Input: part model. Units: mm. Frame: model coordinates. Face numbers are marked on the shaded views. A direction names the side the tool comes from. Round coordinates to 2 decimals unless told otherwise and drop trailing zeros. Write each loop counter-clockwise with the first axis right and the second up, starting at its lowest first coordinate (ties: lowest second). Pieces come first, ordered by that corner, then holes. Notation, with made-up numbers: (-15, 54) - (13, 54) arc R12 ccw to (13, 76) - close; hole circle Ø7 at (52.5, 65). An arc over 180 degrees is marked (long way). One line per item, written item: value. Start each with the question number.
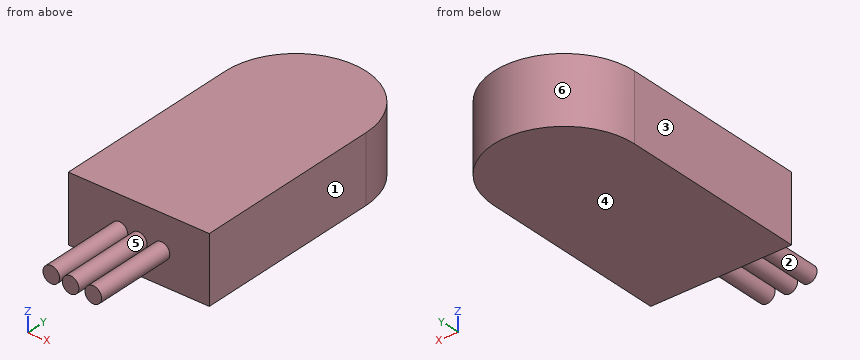
Autodesk Inventor part; units mm, degrees
ref_plane "YZ Plane" through (0, 0, 0) normal (1, 0, 0) x (0, 1, 0)
ref_plane "XZ Plane" through (0, 0, 0) normal (0, 1, 0) x (-1, 0, 0)
ref_plane "XY Plane" through (0, 0, 0) normal (0, 0, 1) x (1, 0, 0)
sketch "Sketch1" plane through (0, 0, 0) normal (0, 0, 1) x (1, 0, 0)
  line L0 (-8.5, 11.5) -> (8.5, 11.5)
  line L1 (8.5, 11.5) -> (8.5, -11.5)
  line L2 (8.5, -11.5) -> (-8.5, -11.5)
  line L3 (-8.5, -11.5) -> (-8.5, 11.5)
  line L4 (-8.5, 11.5) -> (8.5, -11.5) construction
  line L5 (8.5, 11.5) -> (-8.5, -11.5) construction
  arc A0 (8.5, 11.5) -> (-8.5, 11.5) centre (0, 11.5) ccw
  point P0 (0, 0)
  dimension "d0" = 23
  dimension "d1" = 17
extrude "Extrusion1" add sketch "Sketch1" along normal blind 8
sketch "Sketch3" plane through (0, 0, 8) normal (0, 0, 1) x (1, 0, 0)
  line L0 (-8.5, 11.5) -> (-8.5, -11.5)
  line L1 (8.5, -11.5) -> (8.5, 11.5)
  line L2 (-8.5, 11.5) -> (8.5, 11.5)
  point P0 (0, 0)
sketch "Sketch4" plane through (-8.5, -11.5, 0) normal (0, -1, 0) x (1, 0, 0)
  circle A0 centre (6.1706, 4.0145) radius 1
  circle A1 centre (11.2338, 3.8113) radius 1
  circle A2 centre (8.5, 3.8113) radius 1
  point P0 (8.5, 0)
  dimension "d4" = 2
  dimension "d6" = 2
  dimension "d9" = 2
extrude "Extrusion2" add sketch "Sketch4" along normal blind 10 contours A0 | A1
extrude "Extrusion3" add sketch "Sketch4" along normal blind 10 contours A2
properties part number "temperature sensor" material "Rubber, Silicone"
Q1. Cut plane D-D, the plane x = 3. Output: boundary loops of the cut face in (y, z).
Q2. Cut plane B-B, the plane z = 7.5. Output: boundary loops of the cut face in (x, y), and give its area (3 significant figures).
Q3. Material intervals for probe 1 along X at (y, z) = (-16, 4.5); probe 2 along X at (y, z) = (-13.5, 4.25); probe 3 along Z at (x, y) = (0, -20), sorted ascending. Write a range as from..to.
Q4. Cut plane C-C, the plane y = 16. Output: boundary loops of the cut face in (x, z), and give its area (3 significant figures).
Q5. Access query for the marked faces 5 and 6. Directions: +Z, -Z, +X, -X, +Y, -Y. A direction counts if a zero-diameter tool reaches every point of the face in a straight line with its end or side. Return the directions, or none.
Q6. Contact query for flat-ended pins moving along their axis: pin 1 Ø1.5 at (x, z) = (3, 1) entering from -Y; pin 2 Ø1.5 at (x, y) = (-1, -13) entering from +Z; pin 3 Ø4 at (x, z) = (6.5, 2.5) entering from +Y. Output: stop coordinate, or through.
Q7. Cut plane A-A, the plane x = 0. Output: boundary loops of the cut face in (y, z), and give its area (3 significant figures).
Q8. Pull-direction query (X, two-part tool) for the marked faces 1, 2, 3 and 4; classes: pulls with the +X half, pulls with the -X half, needs draft (parallel to the pull), parting line crosses it, or undercut.
A:
1. outline: (-21.5, 2.85) - (-11.5, 2.85) - (-11.5, 0) - (19.45, 0) - (19.45, 8) - (-11.5, 8) - (-11.5, 4.78) - (-21.5, 4.78) - close
2. outline: (-8.5, -11.5) - (8.5, -11.5) - (8.5, 11.5) arc R8.5 ccw to (-8.5, 11.5) - close
2. area: 504 mm²
3. probe 1: x = -3.2..-1.46, -0.73..0.73, 2.01..3.46
3. probe 2: x = -3.3..-1.36, -0.9..0.9, 1.84..3.63
3. probe 3: z = 2.81..4.81
4. outline: (-7.21, 0) - (7.21, 0) - (7.21, 8) - (-7.21, 8) - close
4. area: 115 mm²
5. face 5: -Y
5. face 6: +Z, -Z, +Y
6. pin 1: stops at y = -11.5
6. pin 2: stops at z = 4.83
6. pin 3: stops at y = 18.71
7. outline: (-21.5, 2.81) - (-11.5, 2.81) - (-11.5, 0) - (20, 0) - (20, 8) - (-11.5, 8) - (-11.5, 4.81) - (-21.5, 4.81) - close
7. area: 272 mm²
8. face 1: pulls with the +X half
8. face 2: undercut
8. face 3: pulls with the -X half
8. face 4: needs draft
